from build123d import *
from OCP.BRepFilletAPI import BRepFilletAPI_MakeChamfer

# Parameters (mm, degrees)
BOSS_EXTRUDE1_DEPTH = 0.8
BOSS_EXTRUDE2_DEPTH = 1.3
BOSS_EXTRUDE3_DEPTH = 0.9
BOSS_EXTRUDE3_TAPER = 10
SKETCH4_R           = 1.6
SKETCH4_R_2         = 0.9
BOSS_EXTRUDE4_DEPTH = 2.65
SKETCH5_R           = 0.6
BOSS_EXTRUDE5_DEPTH = 3
CHAMFER1_SIZE       = 0.5
CHAMFER1_SIZE2      = 0.419549816
CHAMFER2_SIZE       = 0.5
SKETCH6_W           = 16.5
SKETCH6_H           = 17.5
BOSS_EXTRUDE6_DEPTH = 4
CHAMFER3_SIZE       = 2.5
CHAMFER4_SIZE       = 2.5
CHAMFER4_SIZE2      = 1.165769145
CHAMFER5_SIZE       = 2.5
CHAMFER5_SIZE2      = 0.669872981


with BuildPart() as part:
    # Sketch1 → Boss-Extrude1 (new body)
    with BuildSketch(Plane(origin=(0, 0, 0), x_dir=(1, 0, 0), z_dir=(0, 1, 0))):
        with BuildLine():
            Line((-6.5, -7.5), (6.5, -7.5))
            ThreePointArc((6.5, -7.5), (7.207106781, -7.207106781), (7.5, -6.5))
            Line((7.5, -6.5), (7.5, 6.5))
            ThreePointArc((7.5, 6.5), (7.207106781, 7.207106781), (6.5, 7.5))
            Line((6.5, 7.5), (-6.5, 7.5))
            ThreePointArc((-6.5, 7.5), (-7.207106781, 7.207106781), (-7.5, 6.5))
            Line((-7.5, 6.5), (-7.5, -6.5))
            ThreePointArc((-7.5, -6.5), (-7.207106781, -7.207106781), (-6.5, -7.5))
        make_face()
    extrude(amount=BOSS_EXTRUDE1_DEPTH)

    # Sketch2 → Boss-Extrude2 (add)
    with BuildSketch(Plane.XZ):
        with BuildLine():
            Line((-6.9, 6.5), (-6.9, -6.5))
            ThreePointArc((-6.9, -6.5), (-6.782842712, -6.782842712), (-6.5, -6.9))
            Line((-6.5, -6.9), (6.5, -6.9))
            ThreePointArc((6.5, -6.9), (6.782842712, -6.782842712), (6.9, -6.5))
            Line((6.9, -6.5), (6.9, 6.5))
            ThreePointArc((6.9, 6.5), (6.782842712, 6.782842712), (6.5, 6.9))
            Line((6.5, 6.9), (-6.5, 6.9))
            ThreePointArc((-6.5, 6.9), (-6.782842712, 6.782842712), (-6.9, 6.5))
        make_face()
    extrude(amount=BOSS_EXTRUDE2_DEPTH)

    # Sketch3 → Boss-Extrude3 (add)
    with BuildSketch(Plane.XZ.offset(1.3)):
        with BuildLine():
            Line((-6.9, 6.5), (-6.9, -6.5))
            ThreePointArc((-6.9, -6.5), (-6.782842712, -6.782842712), (-6.5, -6.9))
            Line((-6.5, -6.9), (6.5, -6.9))
            ThreePointArc((6.5, -6.9), (6.782842712, -6.782842712), (6.9, -6.5))
            Line((6.9, -6.5), (6.9, 6.5))
            ThreePointArc((6.9, 6.5), (6.782842712, 6.782842712), (6.5, 6.9))
            Line((6.5, 6.9), (-6.5, 6.9))
            ThreePointArc((-6.5, 6.9), (-6.782842712, 6.782842712), (-6.9, 6.5))
        make_face()
    extrude(amount=BOSS_EXTRUDE3_DEPTH, taper=BOSS_EXTRUDE3_TAPER)

    # Sketch4 → Boss-Extrude4 (add)
    with BuildSketch(Plane.XZ.offset(2.2)):
        with Locations(Location((0, 0, 0), (0, 0, 270))):
            Circle(SKETCH4_R)
        with Locations(Location((0, -5.5, 0), (0, 0, 270))):
            Circle(SKETCH4_R_2)
        with Locations(Location((0, 5.5, 0), (0, 0, 90))):
            Circle(SKETCH4_R_2)
    extrude(amount=BOSS_EXTRUDE4_DEPTH)

    # Sketch5 → Boss-Extrude5 (add)
    with BuildSketch(Plane.XZ.offset(2.2)):
        with Locations(Location((-5.9, 0, 0), (0, 0, 270))):
            Circle(SKETCH5_R)
        with Locations(Location((-3.8, -5, 0), (0, 0, 270))):
            Circle(SKETCH5_R)
    extrude(amount=BOSS_EXTRUDE5_DEPTH)

    # Chamfer1: one chamfer whose edges measure the first distance from different faces: ONE call of the kernel's chamfer builder (chamfer() names one face for all edges)
    chamfer1_edges_1 = [part.edges().sort_by_distance(p)[0] for p in [
        (-5.9, -5.2, 0.6),
    ]]
    chamfer1_side_1 = [part.faces().sort_by_distance(p)[0] for p in [
        (-5.9, -3.7, 0.6),
    ]]
    chamfer1_edges_2 = [part.edges().sort_by_distance(p)[0] for p in [
        (-3.8, -5.2, -4.4),
    ]]
    chamfer1_side_2 = [part.faces().sort_by_distance(p)[0] for p in [
        (-3.8, -3.7, -4.4),
    ]]
    chamfer1 = BRepFilletAPI_MakeChamfer(part.part.solid().wrapped)
    for e in chamfer1_edges_1:
        chamfer1.Add(CHAMFER1_SIZE, CHAMFER1_SIZE2, e.wrapped, chamfer1_side_1[0].wrapped)  # the first distance lies on this face
    for e in chamfer1_edges_2:
        chamfer1.Add(CHAMFER1_SIZE, CHAMFER1_SIZE2, e.wrapped, chamfer1_side_2[0].wrapped)  # the first distance lies on this face
    add(Compound.cast(chamfer1.Shape()), mode=Mode.REPLACE)

    # Chamfer2
    chamfer2_edges = [part.edges().sort_by_distance(p)[0] for p in [
        (0, -4.85, 1.6),
        (0, -4.85, -4.6),
        (0, -4.85, 4.6),
    ]]
    chamfer(chamfer2_edges, length=CHAMFER2_SIZE)

    # Sketch6 → Boss-Extrude6 (add)
    with BuildSketch(Plane(origin=(0, 0.8, 0), x_dir=(1, 0, 0), z_dir=(0, 1, 0))):
        Rectangle(SKETCH6_W, SKETCH6_H)
    extrude(amount=BOSS_EXTRUDE6_DEPTH)

    # Chamfer3
    chamfer3_edges = [part.edges().sort_by_distance(p)[0] for p in [
        (8.25, 4.8, 0),
    ]]
    chamfer(chamfer3_edges, length=CHAMFER3_SIZE)

    # Chamfer4: one chamfer whose edges measure the first distance from different faces: ONE call of the kernel's chamfer builder (chamfer() names one face for all edges)
    chamfer4_edges_1 = [part.edges().sort_by_distance(p)[0] for p in [
        (-1.25, 4.8, -8.75),
    ]]
    chamfer4_side_1 = [part.faces().sort_by_distance(p)[0] for p in [
        (-0.368621604, 2.742014579, -8.75),
    ]]
    chamfer4_edges_2 = [part.edges().sort_by_distance(p)[0] for p in [
        (-1.25, 4.8, 8.75),
    ]]
    chamfer4_side_2 = [part.faces().sort_by_distance(p)[0] for p in [
        (-0.368621604, 2.742014579, 8.75),
    ]]
    chamfer4 = BRepFilletAPI_MakeChamfer(part.part.solid().wrapped)
    for e in chamfer4_edges_1:
        chamfer4.Add(CHAMFER4_SIZE, CHAMFER4_SIZE2, e.wrapped, chamfer4_side_1[0].wrapped)  # the first distance lies on this face
    for e in chamfer4_edges_2:
        chamfer4.Add(CHAMFER4_SIZE, CHAMFER4_SIZE2, e.wrapped, chamfer4_side_2[0].wrapped)  # the first distance lies on this face
    add(Compound.cast(chamfer4.Shape()), mode=Mode.REPLACE)

    # Chamfer5
    chamfer5_edges = [part.edges().sort_by_distance(p)[0] for p in [
        (-8.25, 4.8, 0),
    ]]
    chamfer5_side = [part.faces().sort_by_distance(p)[0] for p in [
        (-8.25, 2.74931608, 0),
    ]]
    chamfer(chamfer5_edges, length=CHAMFER5_SIZE, length2=CHAMFER5_SIZE2, reference=chamfer5_side[0])


solid = part.part
Input: part model. Units: mm. Frame: model coordinates. A direction names the side the tool comes from. Round coordinates to 2 decimals unless told otherwise and drop trailing zeros. Loops run counter-clockwise (first coordinate to the right, second up) from the corner with the lowest first, then second, coordinate; pieces in that order, holes last. Notation, with made-up numbers: (45, 73.25) -> (79, 73.25) arc R9 ccw to (79, 77.25) -> close; hole circle Ø1 at (61, 44.25). An arc over 180 degrees is marked (long way). Answer as a JSON object with one key per item and string values. Group by question number.
1) Section query B-B on y = 4.25. Output: boundary loops of the cut face in (x, z), plus the area to 3 significant figures.
2) Draft query along X for faces 1 (the cylindrical face through (7.199, 0.394, 7.215)), 2 (the flat face through (0, 2, -8.75)), 3 (the cylindrical face through (-6.486, -3.432, 0.13)). Return one class per face: +X half, -X half, draft (parallel to the pull), parting line (faces both ways), or undercut.
3) Section query A-A on y = -1. Output: boundary loops of the cut face in (x, z).
4) Pin query (flat end, axial travel): pin 1 (1.8 mm diameter, centred on x = 0.5, z = 0.5, fed in from -Y); pin 2 (1.4 mm diameter, centred on y = -1, z = -1.5, fed in from +X); pin 3 (1.4 mm diameter, centred on x = -2, y = -0.5, fed in from +Z). Return the tip coordinate at first contact, or that it passes through.
5) Reachability of faces 4 (the flat face through (-6.9, -1, 0)), 5 (the flat face through (0, -4.85, 0)), 6 (the cylindrical face through (-7.215, 0.394, 7.199)), 7 (the cylindrical face through (0, -3.3, -4.6)) from +Z, -Z, +X, -X, +Y, -Y: full face, straight path, thin tool, end or side. Return the list, or none.
6) Ray query, L1, parallel to Y at x = 3, z = 3.5; L2, parallel to X at y = -0.5, z = 0. Return the intervals inside material, ascending.
Reply:
{
 "1": {"outline": "(-7.73, -7.84) -> (6.3, -7.84) -> (6.3, 7.84) -> (-7.73, 7.84) -> close", "area": "220 mm2"},
 "2": {"face 1": "+X half", "face 2": "draft", "face 3": "undercut"},
 "3": {"outline": "(-6.9, -6.5) arc R0.4 ccw to (-6.5, -6.9) -> (6.5, -6.9) arc R0.4 ccw to (6.9, -6.5) -> (6.9, 6.5) arc R0.4 ccw to (6.5, 6.9) -> (-6.5, 6.9) arc R0.4 ccw to (-6.9, 6.5) -> close"},
 "4": {"pin 1": "stops at y = -4.85", "pin 2": "stops at x = 6.9", "pin 3": "stops at z = 7.5"},
 "5": {"face 4": "+Z, -Z, -X, -Y", "face 5": "+Z, -Z, +X, -Y", "face 6": "+Z, -X, -Y", "face 7": "-Y"},
 "6": {"L1": "y = -2.2 to 4.8", "L2": "x = -6.9 to 6.9"}
}
